The listing builds one solid part. Answer for the finished solid, in the listing's coordinates (mm). A direction names the side the tool comes from. Coordinates: 2 decimals unless noted, no trailing zeros. Order: outer loops, then holes, each group sorted by start corner. A loop starts at its lowest first (then second) coordinate and runs counter-clockwise, first axis right, second up. Notation, with made-up numbers: (89, 59) -> (97, 59) arc R7 cw to (97, 71) -> close; hole circle Ø8 at (0.5, -23.5). An arc over 180 degrees is marked (long way). Write each question's results on one line, items separated by ' | '. Start each with the question number.
(1) The part is cut by section A-A, the plane y = 0. Give the vertices of the cut face in (x, z) (3 decimals).
(2) The part is cut by section D-D, the plane x = -22. Give the vertices of the cut face in (y, z) (3 decimals), then the cut area to 3 significant figures.
(3) A tool of negligible diameter and unlimited length cuts with its end or side. For faces 1 (the face through (-25, 10.16, 0)), 2 (the face through (-4.21, 4.92, 0.54)), 3 (the face through (30.098, 9.798, -0.582)), 4 (the face through (-19, 0, -4.445)), 5 (the face through (-0.2, -4.4, -3.048)), from which of +Z, -Z, +X, -X, +Y, -Y can it reach the whole face along a straight path? Write none if from no direction.
(4) The part is cut by section B-B, the plane x = 22.5. Give the vertices of the cut face in (y, z) (3 decimals), then the cut area to 3 significant figures.
(5) Straight lines are drawn through the part: L1, parallel to Y at x = 0, z = -2.25; L2, parallel to X at y = 0, z = -2.55; L3, parallel to Y at x = 24, z = 3. For each, find the intervals that lie inside material, in ascending order.
(6) Given pin 1 (16.5 mm diameter, centred on x = 2.5, y = -3, fed in from +Z); pin 2 (1.6 mm diameter, centred on x = 7, z = -0.5, fed in from +Y); pin 3 (3 mm diameter, centred on x = -26.5, z = -0.5, fed in from -Y), each flat-ended and moving along its own axis, determine where each tip first touches the part or whether it passes through.
```python
from build123d import *

# Parameters (mm, degrees)
F1_DEPTH     = 3.048
F2_DEPTH     = 4.445
F3_T4_ANGLE  = 205.1460272103
F3_T9_ANGLE  = 205.1460272103
F3_T14_ANGLE = 205.1460272103
F3_T19_ANGLE = 205.1460272103
F4_R         = 1.27
F5_R         = 4.064
F6_DEPTH     = 1.016


# Not quite as in the source:
# - a fillet or chamfer that OpenCascade refuses, or shapes differently, is made with other operations: its cross-section is extruded or revolved along the edge and cut away or added


with BuildPart() as f1:
    # F0 (on Top) → F1 (new body, symmetric)
    with BuildSketch(Plane.XY):
        with BuildLine():
            ThreePointArc((4.1802083301, 9.2602083301), (2.1379760717, 9.932505138), (0, 10.16))
            ThreePointArc((0, 10.16), (-2.1379760717, 9.932505138), (-4.1802083301, 9.2602083301))
            ThreePointArc((-4.1802083301, 9.2602083301), (-10.16, 0), (-4.1802083301, -9.2602083301))
            ThreePointArc((-4.1802083301, -9.2602083301), (0, -10.16), (4.1802083301, -9.2602083301))
            ThreePointArc((4.1802083301, -9.2602083301), (8.5351191156, -5.511564359), (10.16, 0))
            ThreePointArc((10.16, 0), (8.5351191156, 5.511564359), (4.1802083301, 9.2602083301))
        make_face()
        Polygon((-5.7207672085, -4.8174884064), (-7.0324509466, 2.5455855286), (-1.3116837381, 7.3630739349), (0, 6.8882745845), (5.7207672085, 4.8174884064), (7.0324509466, -2.5455855286), (4.5967240587, -4.5967240587), (1.3116837381, -7.3630739349), (0, -6.8882745845), align=None, mode=Mode.SUBTRACT)
    extrude(amount=F1_DEPTH, both=True)

    # F0 (on Top) → F2 (join, symmetric)
    with BuildSketch(Plane.XY):
        with BuildLine():
            ThreePointArc((-4.1802083301, -9.2602083301), (-10.16, 0), (-4.1802083301, 9.2602083301))
            Line((-4.1802083301, 9.2602083301), (-5.08, 10.16))
            Line((-5.08, 10.16), (-10.4775, 10.16))
            ThreePointArc((-10.4775, 10.16), (-15.24, 14.9225), (-20.0025, 10.16))
            Line((-20.0025, 10.16), (-30.48, 10.16))
            Line((-30.48, 10.16), (-30.48, -10.16))
            Line((-30.48, -10.16), (-20.0025, -10.16))
            ThreePointArc((-20.0025, -10.16), (-15.24, -14.9225), (-10.4775, -10.16))
            Line((-10.4775, -10.16), (-5.08, -10.16))
            Line((-5.08, -10.16), (-4.1802083301, -9.2602083301))
        make_face()
        with BuildLine():
            Line((5.08, 10.16), (4.1802083301, 9.2602083301))
            ThreePointArc((4.1802083301, 9.2602083301), (8.5351191156, 5.511564359), (10.16, 0))
            ThreePointArc((10.16, 0), (8.5351191156, -5.511564359), (4.1802083301, -9.2602083301))
            Line((4.1802083301, -9.2602083301), (5.08, -10.16))
            Line((5.08, -10.16), (10.4775, -10.16))
            ThreePointArc((10.4775, -10.16), (15.24, -14.9225), (20.0025, -10.16))
            Line((20.0025, -10.16), (30.48, -10.16))
            Line((30.48, -10.16), (30.48, 10.16))
            Line((30.48, 10.16), (20.0025, 10.16))
            ThreePointArc((20.0025, 10.16), (15.24, 14.9225), (10.4775, 10.16))
            Line((10.4775, 10.16), (5.08, 10.16))
        make_face()
    extrude(amount=F2_DEPTH, both=True)

    # F3: chamfer of 2.54 on 4 edges, made by hand


with BuildPart() as f3_tool2:
    # F3_s3 → F3_t4 (revolve)
    with BuildSketch(Plane(origin=(0, 0, 0), x_dir=(0, 0, 1), z_dir=(0.9760193995, 0.217683559, 0))):
        Polygon((4.445, 12.7), (1.905, 10.16), (4.445, 10.16), align=None)
    revolve(axis=Axis((0, 0, 4.445), (0, 0, -1)), revolution_arc=F3_T4_ANGLE)

    split(bisect_by=Plane.XY.offset(3.048), keep=Keep.TOP)


with BuildPart() as f1_1:
    add(f1.part)

    # F3_t1: cut F3_tool2
    add(f3_tool2.part, mode=Mode.SUBTRACT)


with BuildPart() as f3_tool7:
    # F3_s8 → F3_t9 (revolve)
    with BuildSketch(Plane(origin=(0, 0, 0), x_dir=(0, 0, 1), z_dir=(-0.9760193995, -0.217683559, 0))):
        Polygon((1.905, 10.16), (4.445, 12.7), (4.445, 10.16), align=None)
    revolve(axis=Axis((0, 0, 4.445), (0, 0, -1)), revolution_arc=F3_T9_ANGLE)

    split(bisect_by=Plane.XY.offset(3.048), keep=Keep.TOP)


with BuildPart() as f1_2:
    add(f1_1.part)

    # F3_t6: cut F3_tool7
    add(f3_tool7.part, mode=Mode.SUBTRACT)


with BuildPart() as f3_tool12:
    # F3_s13 → F3_t14 (revolve)
    with BuildSketch(Plane(origin=(0, 0, 0), x_dir=(0, 0, 1), z_dir=(-0.9760193995, -0.217683559, 0))):
        Polygon((-4.445, 12.7), (-1.905, 10.16), (-4.445, 10.16), align=None)
    revolve(axis=Axis((0, 0, -4.445), (0, 0, -1)), revolution_arc=F3_T14_ANGLE)

    split(bisect_by=Plane.XY.offset(-3.048), keep=Keep.BOTTOM)


with BuildPart() as f1_3:
    add(f1_2.part)

    # F3_t11: cut F3_tool12
    add(f3_tool12.part, mode=Mode.SUBTRACT)


with BuildPart() as f3_tool17:
    # F3_s18 → F3_t19 (revolve)
    with BuildSketch(Plane(origin=(0, 0, 0), x_dir=(0, 0, 1), z_dir=(0.9760193995, 0.217683559, 0))):
        Polygon((-1.905, 10.16), (-4.445, 12.7), (-4.445, 10.16), align=None)
    revolve(axis=Axis((0, 0, -4.445), (0, 0, -1)), revolution_arc=F3_T19_ANGLE)

    split(bisect_by=Plane.XY.offset(-3.048), keep=Keep.BOTTOM)


with BuildPart() as f1_4:
    add(f1_3.part)

    # F3_t16: cut F3_tool17
    add(f3_tool17.part, mode=Mode.SUBTRACT)

    # F4
    f4_edges = [f1_4.edges().sort_by_distance(p)[0] for p in [
        (-25.24125, -10.16, 4.445),
        (-30.48, 0, 4.445),
        (-25.24125, 10.16, 4.445),
        (25.24125, -10.16, 4.445),
        (30.48, 0, 4.445),
        (25.24125, 10.16, 4.445),
        (-25.24125, -10.16, -4.445),
        (-30.48, -10.16, 0),
        (25.24125, -10.16, -4.445),
        (30.48, 0, -4.445),
        (30.48, 10.16, 0),
        (-30.48, 10.16, 0),
        (-25.24125, 10.16, -4.445),
        (-30.48, 0, -4.445),
        (-9.04875, 10.16, 4.445),
        (9.04875, 10.16, 4.445),
        (-9.04875, -10.16, 4.445),
        (9.04875, -10.16, 4.445),
        (9.04875, 10.16, -4.445),
        (-9.04875, 10.16, -4.445),
        (-9.04875, -10.16, -4.445),
        (9.04875, -10.16, -4.445),
    ]]
    fillet(f4_edges, radius=F4_R)

    # F5 (on face) → F6 (join)
    with BuildSketch(Plane(origin=(0, 0, -3.048), x_dir=(1, 0, 0), z_dir=(0, 0, -1))):
        with BuildLine():
            ThreePointArc((4.4189755144, -9.4989755144), (8.8332738002, -5.6330413093), (10.4765395251, 0))
            ThreePointArc((10.4765395251, 0), (8.8332738002, 5.6330413093), (4.4189755144, 9.4989755144))
            Line((4.4189755144, 9.4989755144), (4.1802083301, 9.2602083301))
            ThreePointArc((4.1802083301, 9.2602083301), (0, 10.16), (-4.1802083301, 9.2602083301))
            Line((-4.1802083301, 9.2602083301), (-4.4189755144, 9.4989755144))
            ThreePointArc((-4.4189755144, 9.4989755144), (-10.4765395251, 0), (-4.4189755144, -9.4989755144))
            Line((-4.4189755144, -9.4989755144), (-4.1802083301, -9.2602083301))
            ThreePointArc((-4.1802083301, -9.2602083301), (0, -10.16), (4.1802083301, -9.2602083301))
            Line((4.1802083301, -9.2602083301), (4.4189755144, -9.4989755144))
        make_face()
        Polygon((-1.3116837381, -7.3630739349), (-7.0324509466, -2.5455855286), (-5.7207672085, 4.8174884064), (1.3116837381, 7.3630739349), (7.0324509466, 2.5455855286), (5.7207672085, -4.8174884064), align=None, mode=Mode.SUBTRACT)
        Polygon((-5.7207672085, 4.8174884064), (-7.0324509466, -2.5455855286), (-1.3116837381, -7.3630739349), (5.7207672085, -4.8174884064), (7.0324509466, 2.5455855286), (1.3116837381, 7.3630739349), align=None)
        Circle(F5_R, mode=Mode.SUBTRACT)
    extrude(amount=-F6_DEPTH)


solid = f1_4.part
```
Established:
1) outline: (-30.48, -3.175) arc R1.27 ccw to (-29.21, -4.445) -> (-12.7, -4.445) -> (-11.303, -3.048) -> (-4.064, -3.048) -> (-4.064, -2.032) -> (-6.579, -2.032) -> (-6.579, 3.048) -> (-11.303, 3.048) -> (-12.7, 4.445) -> (-29.21, 4.445) arc R1.27 ccw to (-30.48, 3.175) -> close; (4.064, -3.048) -> (11.303, -3.048) -> (12.7, -4.445) -> (29.21, -4.445) arc R1.27 ccw to (30.48, -3.175) -> (30.48, 3.175) arc R1.27 ccw to (29.21, 4.445) -> (12.7, 4.445) -> (11.303, 3.048) -> (6.579, 3.048) -> (6.579, -2.032) -> (4.064, -2.032) -> close
2) outline: (-10.16, -3.175) arc R1.27 ccw to (-8.89, -4.445) -> (8.89, -4.445) arc R1.27 ccw to (10.16, -3.175) -> (10.16, 3.175) arc R1.27 ccw to (8.89, 4.445) -> (-8.89, 4.445) arc R1.27 ccw to (-10.16, 3.175) -> close | area: 179 mm^2
3) face 1: +Z, -Z, -X, +Y | face 2: +Z | face 3: +Z, -Z, +X, +Y | face 4: -Z, +X, -X, +Y, -Y | face 5: -Z
4) outline: (-10.16, -3.175) arc R1.27 ccw to (-8.89, -4.445) -> (10.16, -4.445) -> (10.16, 3.175) arc R1.27 ccw to (8.89, 4.445) -> (-8.89, 4.445) arc R1.27 ccw to (-10.16, 3.175) -> close | area: 180 mm^2
5) L1: y = -10.16 to -4.06, 4.06 to 10.16 | L2: x = -30.48 to -4.06, 4.06 to 30.48 | L3: y = -10.16 to 10.16
6) pin 1: stops at z = 3.9 | pin 2: stops at y = 10.16 | pin 3: stops at y = -10.16
